The figure shows three views and two pictorial views of one solid part (mm, origin at its lowest corner). Answer the questions. A direction names the side the tool comes from. Coordinates: 2 decimals unless noted, no trailing zeros. Loops run counter-clockwise (first coordinate to the right, second up) from the corner with the lowest first, then second, coordinate; pieces in that order, holes last.
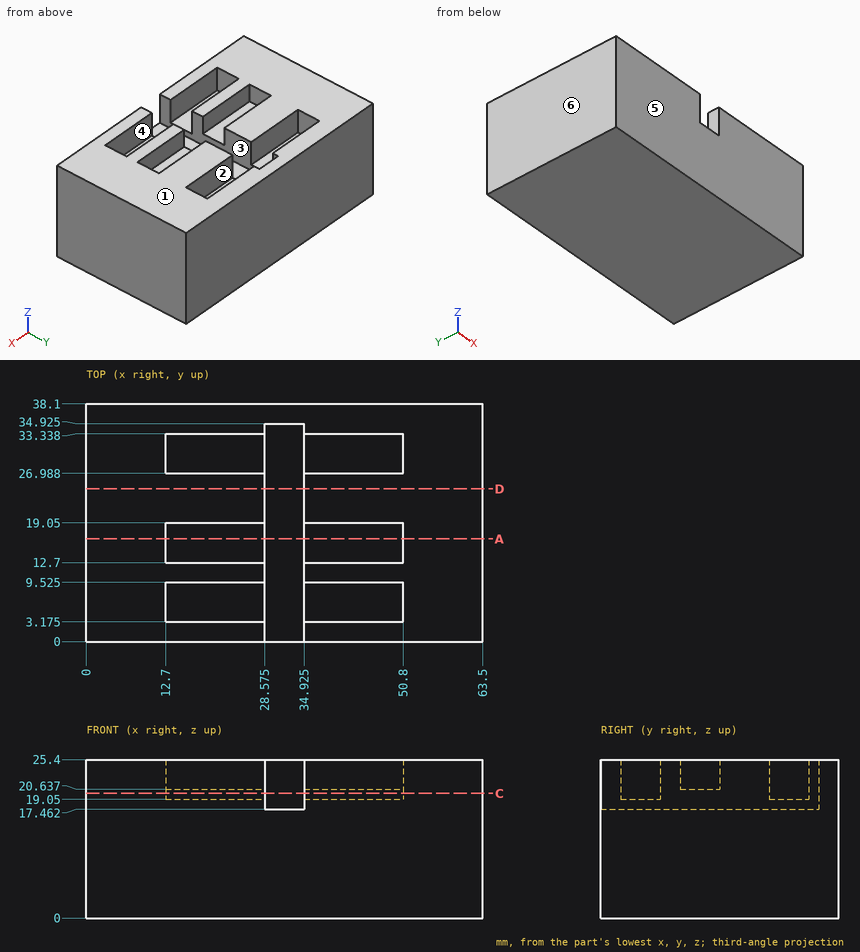
1. Straight lines are drawn through the part: probe 1 along X at (y, z) = (21, 18.25) (1 decimal); probe 2 along X at (y, z) = (7, 24.25); probe 3 along Z at (x, y) = (39.5, 27.5). For each, find the intervals that lie inside material, in ascending order.
2. A cutting plane is placed at A-A, the plane y = 16.5. Give the vertices of the cut face in (x, z) (1 decimal), then the cut area to 3 significant figures.
3. A cutting plane is placed at D-D, the plane y = 24.5. Give the vertices of the cut face in (x, z) (1 decimal).
4. For the marked faces 1, 2 and 3, determine the directions among +Z, -Z, +X, -X, +Y, -Y from which every point of the face is accessible in a straight line to the end or side of a thin tool.
5. A cutting plane is placed at C-C, the plane z = 20. Give the vertices of the cut face in (x, y) (1 decimal), then the cut area to 3 significant figures.
6. Each of these flat-tipped pins is pushed along its axis until it touches: P1, Ø5, axis at x = 23, y = 30, coming from the +Z side; P2, Ø1.9, axis at x = 17, y = 16, coming from the +Z side; P3, Ø3, axis at x = 31.5, y = 26, coming from the +Z side. Where does it stop, or does it pass through?
7. Determine the mould class of the marked faces 4, 5 and 6 for opening direction Y: released by +Y, released by -Y, zero draft, split by the parting line, or undercut.
Answers below:
1. probe 1: x = 0 to 28.6, 34.9 to 63.5
1. probe 2: x = 0 to 12.7, 50.8 to 63.5
1. probe 3: z = 0 to 19.05
2. outline: (0, 0) - (63.5, 0) - (63.5, 25.4) - (50.8, 25.4) - (50.8, 20.6) - (34.9, 20.6) - (34.9, 17.5) - (28.6, 17.5) - (28.6, 20.6) - (12.7, 20.6) - (12.7, 25.4) - (0, 25.4) - close
2. area: 1,410 mm2
3. outline: (0, 0) - (63.5, 0) - (63.5, 25.4) - (34.9, 25.4) - (34.9, 17.5) - (28.6, 17.5) - (28.6, 25.4) - (0, 25.4) - close
4. face 1: +Z, +X, -X, +Y, -Y
4. face 2: +Z
4. face 3: +Z, -Y
5. outline: (0, 0) - (28.6, 0) - (28.6, 3.2) - (12.7, 3.2) - (12.7, 9.5) - (28.6, 9.5) - (28.6, 27) - (12.7, 27) - (12.7, 33.3) - (28.6, 33.3) - (28.6, 34.9) - (34.9, 34.9) - (34.9, 33.3) - (50.8, 33.3) - (50.8, 27) - (34.9, 27) - (34.9, 9.5) - (50.8, 9.5) - (50.8, 3.2) - (34.9, 3.2) - (34.9, 0) - (63.5, 0) - (63.5, 38.1) - (0, 38.1) - close
5. area: 1,790 mm2
6. P1: stops at z = 19.05
6. P2: stops at z = 20.64
6. P3: stops at z = 17.46
7. face 4: undercut
7. face 5: released by -Y
7. face 6: zero draft
